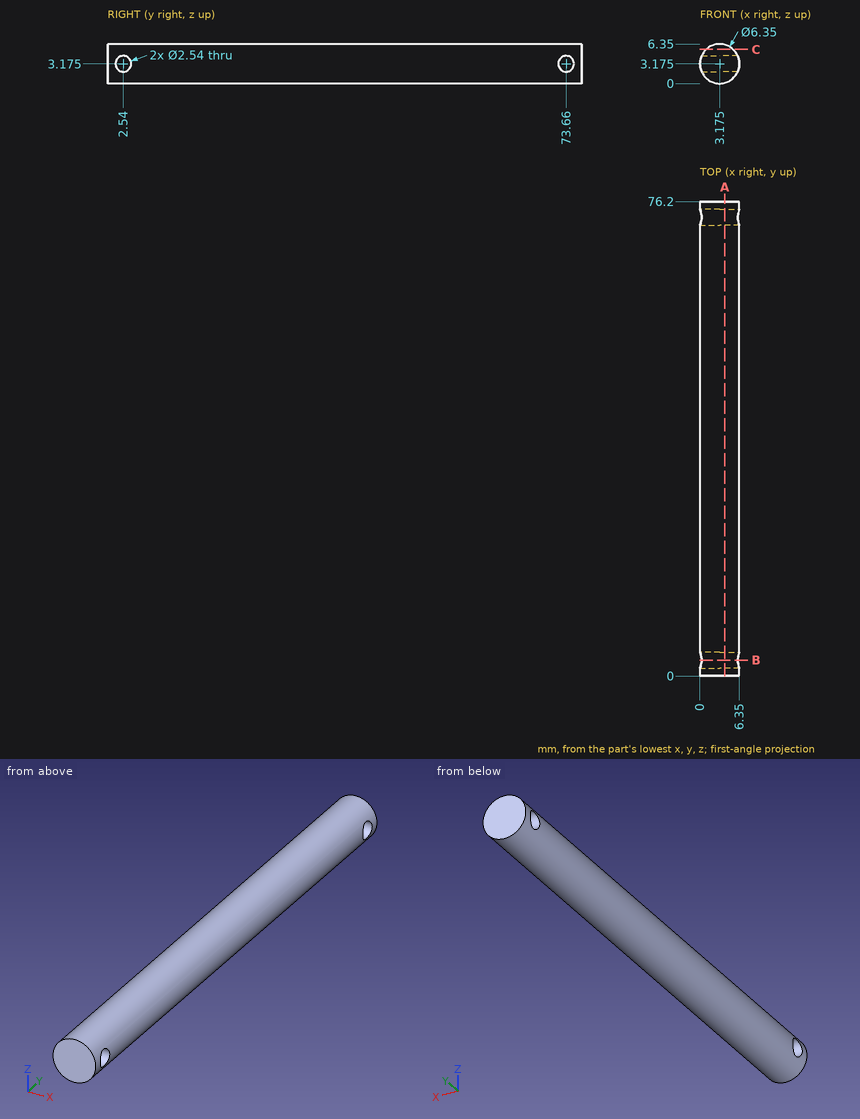
Drawing for the job (mm, zero at the part's lowest x, y, z). Give positions to 0.01 mm unless a question says otherwise; leave off trailing zeros. Order: outer loops, then holes, each group sorted by start corner. A loop starts at its lowest first (then second) coordinate and runs counter-clockwise, first axis right, second up. Notation, with made-up numbers: M -24,-33 L -17,-33 A12 ccw -17,-14 Z; hole C 70.25,76 d7. An arc over 180 degrees is marked long. Put each result on its own line as item: value.
Item 1: Slice it at B-B, the plane y = 2.54. Write the cut outline in (x, z) (3 decimals), plus the area to 3 significant figures.
From the geometry:
outline: M 0.265,1.905 A3.175 ccw 6.085,1.905 Z; M 0.265,4.445 L 6.085,4.445 A3.175 ccw Z
area: 16.0 mm2
Item 2: Slice it at A-A, the plane x = 4. Write the cut outline in (y, z) (3 decimals), plus the area to 3 significant figures.
From the geometry:
outline: M 0,0.109 L 76.2,0.109 L 76.2,6.241 L 0,6.241 Z; hole C 2.54,3.175 d2.54; hole C 73.66,3.175 d2.54
area: 457 mm2
Item 3: Flat gauge pins, fed straight in: pin 1 Ø3 at (y, z) = (43.5, 5.5) entering from +X; pin 2 Ø2 at (y, z) = (59, 1) entering from +X; pin 3 Ø3 at (x, y) = (5, 44) entering from +Z. Where does each tip first touch, or does it go through?
From the geometry:
pin 1: stops at x = 6.24
pin 2: stops at x = 6.12
pin 3: stops at z = 6.33
Item 4: Probe line 1 (Y direction, x = 5, z = 3.25); line 2 (Y direction, x = 6, z = 2.75); line 3 (Z direction, x = 3.25, y = 60.5). List the from-to ranges inside material, lowest first. Write a range as [from, to].
From the geometry:
line 1: y = [0, 1.27], [3.81, 72.39], [74.93, 76.2]
line 2: y = [0, 1.34], [3.74, 72.46], [74.86, 76.2]
line 3: z = [0, 6.35]
Item 5: Slice it at C-C, the plane z = 5.5. Write the cut outline in (x, y).
From the geometry:
outline: M 1.01,0 L 5.34,0 L 5.34,76.2 L 1.01,76.2 Z
